Here's how the part is built. I have some questions about the finished solid (model axes, mm). A direction names the side the tool comes from. Give positions to 0.01 mm unless a question says otherwise; leave off trailing zeros. Order: outer loops, then holes, each group sorted by start corner. A loop starts at its lowest first (then second) coordinate and runs counter-clockwise, first axis right, second up.
from build123d import *

# Parameters (mm, degrees)
F1_DEPTH = 76.2
F1_TAPER = -3
F2_R     = 11.2646539413
F3_DEPTH = 127
F4_T     = -12.7
F5_D     = 6.35
F6_W     = 14.6276317537
F6_H     = 52.8245866299
F8_DEPTH = 38.1


with BuildPart() as f1:
    # F0 (on Top) → F1 (new body)
    with BuildSketch(Plane.XY):
        Polygon((0, 0), (-97.3766073585, 8.691851981), (-91.719087719, -33.0650627753), (6.7379414104, -41.8533533812), align=None)
    extrude(amount=F1_DEPTH, taper=F1_TAPER)

    # F2 (on face) → F3 (cut)
    with BuildSketch(Plane(origin=(-94.2061631176, -12.7637116177, -4.9822445688), x_dir=(0.1338892143, -0.9909710079, 0.0070809466), z_dir=(-0.9895880386, -0.1340763271, -0.0523359562))):
        with Locations((-5.5252215825, 44.5609055459)):
            Circle(F2_R)
    extrude(amount=-F3_DEPTH, mode=Mode.SUBTRACT)

    # F4
    f4_openings = [f1.faces().sort_by_distance(p)[0] for p in [
        (-45.58374, -16.595081, 0),
    ]]
    offset(amount=F4_T, openings=f4_openings)

    # F5 (through all)
    with Locations(Plane(origin=(-3.6430423813, -40.8137538844, -2.1474622433), x_dir=(0.9960508275, -0.088662203, -0.004665063), z_dir=(-0.088784847, -0.9946749211, -0.0523359562))):
        with Locations((-54.7213628888, 39.8817788885)):
            Hole(F5_D / 2)

    # F6 (on face) → F8 (join)
    with BuildSketch(Plane(origin=(-3.6430423813, -40.8137538844, -2.1474622433), x_dir=(0.9960508275, -0.088662203, -0.004665063), z_dir=(-0.088784847, -0.9946749211, -0.0523359562))):
        with Locations((-36.151945591, 32.273888588)):
            Rectangle(F6_W, F6_H)
    extrude(amount=F8_DEPTH)


solid = f1.part
Q1. For faces 4 (the face through (-43.97, -23.97, 38.52)), 5 (the face through (-45, -17, 76.2)), which set-ups out of +Z, -Z, +X, -X, +Y, -Y let a thin tool reach every point of the face, with its end or its side?
Filled sheet:
face 4: none
face 5: +Z, +X, -X, +Y, -Y
Q2. I'm going to push flat-ended pins straight in: P1, Ø12, axis at x = -51.5, z = 50, coming from the +Y side; P2, Ø10, axis at x = -48, z = 62.5, coming from the +Y side; P3, Ø12, axis at x = -29.5, y = -11, coming from the -Z side; P4, Ø12, axis at y = -21.5, z = 28.5, coming from the -X side. Where does each tip first touch, or does it pass through?
Filled sheet:
P1: stops at y = 7.85
P2: stops at y = 8.09
P3: stops at z = 0
P4: stops at x = -95.67
Q3. I need wall thicknesses on L1, parallel to Y at x = -17, z = 53; L2, parallel to Y at x = -54, z = 9.5; L3, parallel to Z at x = -32.5, y = 0.5. Which ranges of each line are inside material? Lowest first, please.
Filled sheet:
L1: y = -42.52 to -29.76, -18.65 to -2.81
L2: y = -36.93 to -24.16, -7.45 to 5.32
L3: z = 0 to 31.66, 54.13 to 76.2
Q4. If we section it at A-A on y = -61.5: List the corners of the cut face in (x, z) for me.
Filled sheet:
outline: (-49.1, 2.63) - (-34.41, 2.63) - (-34.17, 55.53) - (-48.85, 55.53) - close
Q5. Thinking about a two-plate mould opening in Y: for faces 1 (the face through (-45, -26, 0)), 2 (the face through (-43.14, -77.21, 28.63)), 3 (the face through (-57.891, -12.767, 44.95)), which applies, released by +Y, released by -Y, zero draft, split by the parting line, or undercut?
Filled sheet:
face 1: zero draft
face 2: released by -Y
face 3: undercut
